Design review of the part built by this model. Coordinates are the model's own, in mm. A direction names the side the tool comes from. Coordinates: 2 decimals unless noted, no trailing zeros. Order: outer loops, then holes, each group sorted by start corner. A loop starts at its lowest first (then second) coordinate and runs counter-clockwise, first axis right, second up. Notation, with made-up numbers: M 56.5,74.25 L 83.5,74.25 A10 cw 83.5,92.25 Z; hole C 34.5,45 d5. An arc over 180 degrees is marked long. Use CSV: the item, a comma, the result in double quotes.
```python
from build123d import *

# Parameters (mm, degrees)
F0_R          = 4.7625
F1_DEPTH      = 1079.5
F3_R          = 3.937
F4_DEPTH      = 12.7
F4_DEPTH_BACK = 12.7
F5_W          = 19.05
F5_H          = 60.4399840052
F6_DEPTH      = 84.921


# Not quite as in the source:
# - a feature names something its author has since deleted; it is built from what else it names


with BuildPart() as f1:
    # F0 (on Right) → F1 (new body)
    with BuildSketch(Plane.YZ):
        with BuildLine():
            Line((-11.938, 0), (0, 0))
            Line((0, 0), (0, -3.048))
            Line((0, -3.048), (0, -8.6186548987))
            Line((0, -8.6186548987), (0, -75.9830698371))
            Line((0, -75.9830698371), (3.302, -75.9830698371))
            Line((3.302, -75.9830698371), (3.302, -8.6186548987))
            ThreePointArc((3.302, -8.6186548987), (12.5020792667, -4.6210291468), (6.35, 3.302))
            Line((6.35, 3.302), (-88.9, 3.302))
            Line((-88.9, 3.302), (-88.9, 0))
            Line((-88.9, 0), (-76.962, 0))
            Line((-76.962, 0), (-64.3, 0))
            Line((-64.3, 0), (-64.3, -6.35))
            ThreePointArc((-64.3, -6.35), (-82.2605122421, -13.7894877579), (-89.7, -31.75))
            Line((-89.7, -31.75), (-89.7, -96.35))
            Line((-89.7, -96.35), (-12.7, -96.35))
            Line((-12.7, -96.35), (-12.7, -31.75))
            ThreePointArc((-12.7, -31.75), (-20.1394877579, -13.7894877579), (-38.1, -6.35))
            Line((-38.1, -6.35), (-54.3371811509, -6.35))
            Line((-54.3371811509, -6.35), (-54.3371811509, 0))
            Line((-54.3371811509, 0), (-11.938, 0))
        make_face()
        with Locations((6.35, -3.048)):
            Circle(F0_R, mode=Mode.SUBTRACT)
    extrude(amount=F1_DEPTH)

    # F3 (on offset) → F4 (join, two sides)
    with BuildSketch(Plane.YZ.offset(539.75)) as f4_sk:
        with BuildLine():
            Line((3.302, -11.43), (3.302, -68.58))
            Line((3.302, -68.58), (17.5895, -68.58))
            Line((17.5895, -68.58), (46.489693531, -23.6623454656))
            ThreePointArc((46.489693531, -23.6623454656), (46.7820764127, -15.5652920647), (39.8145, -11.43))
            Line((39.8145, -11.43), (3.302, -11.43))
        make_face()
        with Locations((39.8145, -19.3675)):
            Circle(F3_R, mode=Mode.SUBTRACT)
    extrude(amount=F4_DEPTH)
    extrude(f4_sk.sketch, amount=-F4_DEPTH_BACK)

    # F5 (on face) → F6 (cut, through all)
    with BuildSketch(Plane.XY.offset(-11.43)):
        with Locations((539.75, 36.6969920026)):
            Rectangle(F5_W, F5_H)
    extrude(amount=-F6_DEPTH, mode=Mode.SUBTRACT)


solid = f1.part
```
(1) Add section B-B on y = -22. State the section outline as (x, z) points.
The answers:
outline,"M 0,-96.35 L 1079.5,-96.35 L 1079.5,-12.1 L 0,-12.1 Z; M 0,0 L 1079.5,0 L 1079.5,3.3 L 0,3.3 Z"
(2) Wall thickness on probe 1 along Y at (x, z) = (280.5, -65); probe 2 along Z at (x, y) = (901.5, -41.5); probe 3 along Z at (x, y) = (362, -79.5): over which ranges is each line inside the solid? List them lowest first.
The answers:
probe 1,"y = -89.7 to -12.7, 0 to 3.3"
probe 2,"z = -96.35 to -6.35, 0 to 3.3"
probe 3,"z = -96.35 to -11.4, 0 to 3.3"
(3) For faces 5 (the face through (552.45, 20, -33)), 6 (the face through (532, 0, -37)), 7 (the face through (527.05, 20, -33)), 8 (the face through (530.225, 22, -33)), 9 (the face through (532, -77, 0)), list the 3-axis set-ups (+Z, -Z, +X, -X, +Y, -Y) from which the entire face can be reached by the end or side of a thin tool; tool diameter is ignored.
The answers:
face 5,"-Z, +X, +Y"
face 6,"-Z, +X, -X"
face 7,"-Z, -X, +Y"
face 8,"-Z, +Y"
face 9,"+X, -X, -Y"
(4) Clearance check with flat-ended pins moving along their axes: P1, Ø2.5, axis at x = 314.5, y = 2, coming from the -Z side; P2, Ø5.5, axis at x = 541.5, z = -30.5, coming from the +Y side; P3, Ø10, axis at y = 21, z = -50.5, coming from the +X side; P4, Ø7, axis at y = 39.81, z = -19.37, coming from the +X side. State where each tip first meets the part, or that it passes through.
The answers:
P1,"stops at z = -75.98"
P2,"stops at y = 6.48"
P3,"stops at x = 552.45"
P4,"passes through"
(5) Add section A-A on z = -57. State the section outline as (x, y) points (3 decimals).
The answers:
outline,"M 0,-89.7 L 1079.5,-89.7 L 1079.5,-12.7 L 0,-12.7 Z; M 0,0 L 1079.5,0 L 1079.5,3.302 L 552.45,3.302 L 552.45,25.04 L 549.275,25.04 L 549.275,6.477 L 530.225,6.477 L 530.225,25.04 L 527.05,25.04 L 527.05,3.302 L 0,3.302 Z"
(6) The part is to be moulded in two halves that separate along Z. For faces 1 (the face through (532, -28, 0)), 2 (the face through (549.275, 22, -33)), 3 (the face through (532, -41, 3.302)), 4 (the face through (532.19, -82.06, -13.59)), say which applies: pulls with the +Z half, pulls with the -Z half, needs draft (parallel to the pull), parting line crosses it, or undercut.
The answers:
face 1,"undercut"
face 2,"needs draft"
face 3,"pulls with the +Z half"
face 4,"undercut"
